Input: dimensioned drawing with shaded views. Units: mm. Origin: part minimum x, y, z. Coordinates: 2 decimals unless noted, no trailing zeros. Write each loop counter-clockwise with the first axis right and the second up, starting at its lowest first coordinate (ties: lowest second). Pieces come first, ordered by that corner, then holes. Notation, with made-up numbers: (-35, -33) -> (21, -33) arc R35 cw to (21, -1) -> close; hole circle Ø3 at (78, -18.5). An arc over 180 degrees is marked (long way). One line per item, written item: value. Start each with the question number.
1. Line query: line 1 (Y direction, x = 10, z = 12.7) (3 decimals); line 2 (Z direction, x = 12.25, y = 14); line 3 (Z direction, x = 7.75, y = 12). Output: solid intervals per line, ascending.
2. Mould query, pull axis Y, two halves, no side actions, for the marked faces 1, 2 and 3. Classes: released by +Y, released by -Y, zero draft, split by the parting line, or undercut.
3. First-contact query: P1, Ø7.5, axis at y = 12.7, z = 12.7, coming from the +X side; P2, Ø1, axis at x = 6.5, y = 6.5, coming from the +Z side; P3, Ø2, axis at x = 7.5, y = 15, coming from the -Z side. Flat tips, straight axial feed; report the tip coordinate or a pass-through.
4. Section query C-C, the plane y = 4.5. Output: boundary loops of the cut face in (x, z), and give its area (3 significant figures).
5. Section query A-A, the plane y = 12.7. Output: boundary loops of the cut face in (x, z) (3 decimals), and give its area (3 significant figures).
6. Section query B-B, the plane x = 11. Output: boundary loops of the cut face in (y, z) (3 decimals).
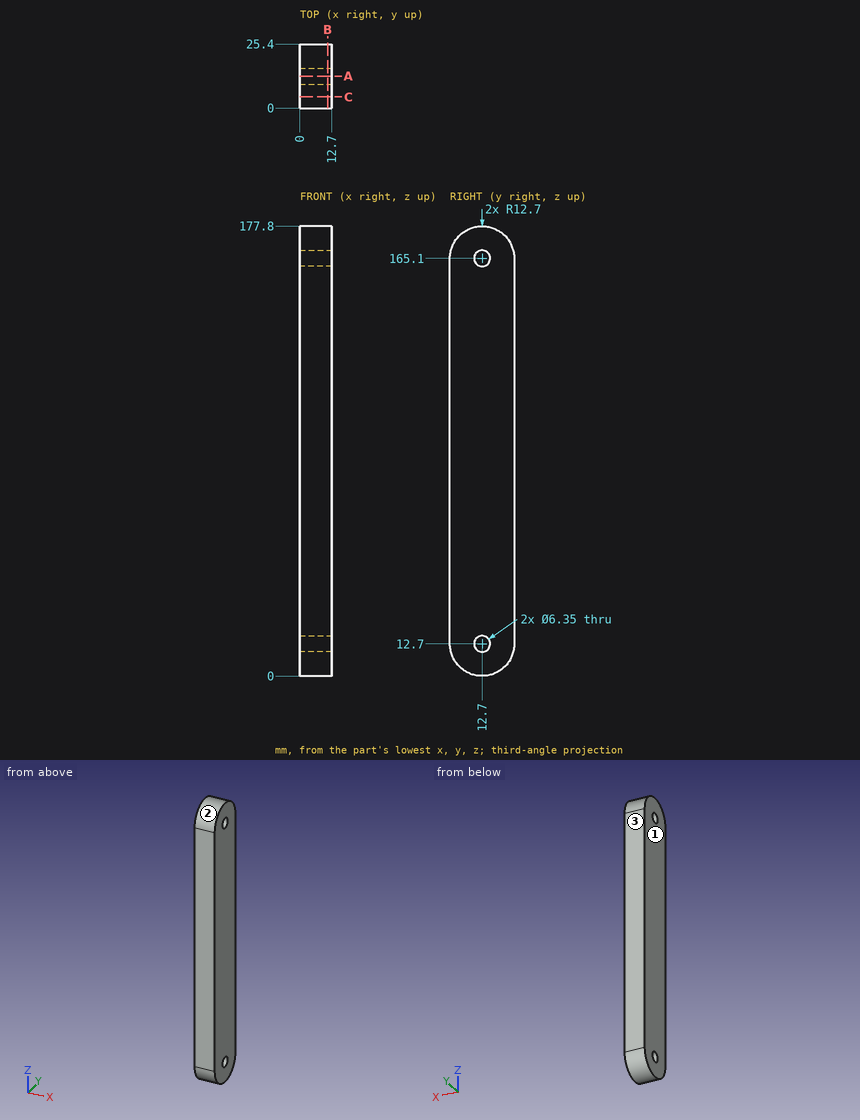
Computed values:
1. line 1: y = 0 to 9.525, 15.875 to 25.4
1. line 2: z = 0.07 to 9.8, 15.6 to 162.2, 168 to 177.73
1. line 3: z = 0.02 to 9.6, 15.8 to 162, 168.2 to 177.78
2. face 1: zero draft
2. face 2: split by the parting line
2. face 3: released by +Y
3. P1: stops at x = 12.7
3. P2: stops at z = 176.45
3. P3: stops at z = 0.07
4. outline: (0, 3) -> (12.7, 3) -> (12.7, 174.8) -> (0, 174.8) -> close
4. area: 2,180 mm²
5. outline: (0, 0) -> (12.7, 0) -> (12.7, 9.525) -> (0, 9.525) -> close; (0, 15.875) -> (12.7, 15.875) -> (12.7, 161.925) -> (0, 161.925) -> close; (0, 168.275) -> (12.7, 168.275) -> (12.7, 177.8) -> (0, 177.8) -> close
5. area: 2,100 mm²
6. outline: (0, 12.7) arc R12.7 ccw to (25.4, 12.7) -> (25.4, 165.1) arc R12.7 ccw to (0, 165.1) -> close; hole circle Ø6.35 at (12.7, 12.7); hole circle Ø6.35 at (12.7, 165.1)
